Check sheet for the modelled part. Datum: model origin and axes. Units: mm. A direction names the side the tool comes from. Coordinates: 2 decimals unless noted, no trailing zeros. Loops run counter-clockwise (first coordinate to the right, second up) from the corner with the lowest first, then second, coordinate; pieces in that order, holes last.
```python
from build123d import *

# Parameters (mm, degrees)
SKETCH1_R           = 10
BOSS_EXTRUDE1_DEPTH = 25
SKETCH4_R           = 1.5
BOSS_EXTRUDE2_DEPTH = 20
CUT_EXTRUDE2_DEPTH  = 29.722813233
SKETCH6_W           = 6.24870068
SKETCH6_H           = 3
BOSS_EXTRUDE3_DEPTH = 25
SKETCH7_R           = 1.75
CUT_EXTRUDE3_DEPTH  = 30.983328701


# Read off the part's stored shape, not the designer's step: Boundary-Cut1
with BuildPart() as part:
    # Sketch1 → Boss-Extrude1 (new body)
    with BuildSketch(Plane(origin=(0, 0, 0), x_dir=(1, 0, 0), z_dir=(0, 1, 0))):
        with Locations(Location((0, 0, 0), (0, 0, 270))):
            Circle(SKETCH1_R)
    extrude(amount=BOSS_EXTRUDE1_DEPTH)

    # Boundary-Cut1 outline → Boundary-Cut1 (revolve, cut)
    with BuildSketch(Plane.XY):
        Polygon((0, 5), (5, 5), (6.5, 25), (0, 25), align=None)
    revolve(axis=Axis((0, 0, 0), (0, 1, 0)), mode=Mode.SUBTRACT)

    # Sketch4 → Boss-Extrude2 (add)
    with BuildSketch(Plane(origin=(0, 5, 0), x_dir=(1, 0, 0), z_dir=(0, 1, 0))):
        with Locations(Location((0, 0, 0), (0, 0, 90))):
            Circle(SKETCH4_R)
    extrude(amount=BOSS_EXTRUDE2_DEPTH)

    # Sketch5 → Cut-Extrude2 (cut, through all)
    with BuildSketch(Plane(origin=(0, 25, 0), x_dir=(1, 0, 0), z_dir=(0, 1, 0))):
        with BuildLine():
            Line((-10, 0), (-1.5, 0))
            ThreePointArc((-1.5, 0), (0, 1.5), (1.5, 0))
            Line((1.5, 0), (10, 0))
            ThreePointArc((10, 0), (0, -10), (-10, 0))
        make_face()
    extrude(amount=-CUT_EXTRUDE2_DEPTH, mode=Mode.SUBTRACT)

    # Sketch6 → Boss-Extrude3 (add)
    with BuildSketch(Plane(origin=(0, 0, 0), x_dir=(1, 0, 0), z_dir=(0, 1, 0))):
        with Locations((-11.87564966, 1.5)):
            Rectangle(SKETCH6_W, SKETCH6_H)
    boss_extrude3 = extrude(amount=BOSS_EXTRUDE3_DEPTH)

    # Sketch7 → Cut-Extrude3 (cut, through all)
    with BuildSketch(Plane(origin=(0, 0, -3), x_dir=(-1, 0, 0), z_dir=(0, 0, -1))):
        with Locations((12.269696007, 5)):
            Circle(SKETCH7_R)
        with Locations((12.269696007, 20)):
            Circle(SKETCH7_R)
    cut_extrude3 = extrude(amount=-CUT_EXTRUDE3_DEPTH, mode=Mode.SUBTRACT)

    # Mirror1: Boss-Extrude3, Cut-Extrude3 across plane
    add(boss_extrude3.mirror(Plane(origin=(0, 0, 0), x_dir=(0, 0, 1), z_dir=(1, 0, 0))))
    add(cut_extrude3.mirror(Plane(origin=(0, 0, 0), x_dir=(0, 0, 1), z_dir=(1, 0, 0))), mode=Mode.SUBTRACT)


solid = part.part
```
1) Section check B-B on x = 0. Enter the section's corners in (y, z).
Answer sheet:
outline: (0, -10) - (25, -10) - (25, -6.5) - (5, -5) - (5, -1.5) - (0, -1.5) - close
2) Set-up check for faces 1 (the flat face through (-12, 12, -3)), 2 (the flat face through (0, 5, -3)), 3 (the cylindrical face through (11.89, 3.29, -1.52)), 4 (the flat face through (12, 12, -3)): record each of +Z, -Z, +X, -X, +Y, -Y from which the full face is reachable in a straight line by a thin tool's end or side.
Answer sheet:
face 1: -Z, -X, +Y, -Y
face 2: +Z, +Y
face 3: +Z, -Z
face 4: -Z, +X, +Y, -Y
3) Section check A-A on y = 20. Enter the section's corners in (x, z) (3 decimals).
Answer sheet:
outline: (-15, -3) - (-14.02, -3) - (-14.02, 0) - (-15, 0) - close; (-10.52, -3) - (-9.539, -3) arc R10 ccw to (9.539, -3) - (10.52, -3) - (10.52, 0) - (6.125, 0) arc R6.125 cw to (-6.125, 0) - (-10.52, 0) - close; (14.02, -3) - (15, -3) - (15, 0) - (14.02, 0) - close
4) Mould release check, pull along Y, two halves, no side actions. Record for faces 5 (the cylindrical face through (0, 2.5, -1.5)), 6 (the cylindrical face through (12.042, 21.735, -1.521)), 7 (the flat face through (0, 25, -7)): +Y half, -Y half, draft (parallel to the pull), parting line (faces both ways), or undercut.
Answer sheet:
face 5: draft
face 6: undercut
face 7: +Y half
5) Section check D-D on y = 7.75. Enter the section's corners in (x, z).
Answer sheet:
outline: (-15, -3) - (-9.54, -3) arc R10 ccw to (9.54, -3) - (15, -3) - (15, 0) - (5.21, 0) arc R5.21 cw to (-5.21, 0) - (-15, 0) - close
6) Depth check by flat-ended pin: pin 1 (4.5 mm diameter, centred on x = 13, y = 15, fed in from -Z); pin 2 (3 mm diameter, centred on y = 8, z = -5, fed in from +X); pin 3 (1.5 mm diameter, centred on y = 12.5, z = -8, fed in from +X). Enter the tip coordinate at first touch or a pass-through.
Answer sheet:
pin 1: stops at z = -3
pin 2: stops at x = 9.37
pin 3: stops at x = 6.89
7) Scan lines: line 1 (X direction, y = 4.5, z = -1); line 2 (X direction, y = 18.5, z = -1); line 3 (Z direction, x = -13, y = 9.5). Record each from-to range of solid material in increasing order.
Answer sheet:
line 1: x = -15 to -13.95, -10.59 to -1.12, 1.12 to 10.59, 13.95 to 15
line 2: x = -15 to -13.17, -11.37 to -5.93, 5.93 to 11.37, 13.17 to 15
line 3: z = -3 to 0
8) Section check C-C on z = -0.75. Give the number of separate pieces and of enclosed holes in the cut face, plus the area to 3 significant figures.
Answer sheet:
separate pieces: 2
enclosed holes: 4
area: 471 mm2
